from build123d import *

# Parameters (mm, degrees)
F1_DEPTH = 40.386
F2_R     = 15.605309
F3_DEPTH = 61.976


with BuildPart() as f1:
    # F0 (on Top) → F1 (new body)
    with BuildSketch(Plane.XY):
        Polygon((78.89688, 0), (-75.812049, 0), (-75.812049, -32.37997), (78.89688, -38.405467), align=None)
    extrude(amount=F1_DEPTH)

    # F2 (on face) → F3 (join)
    with BuildSketch(Plane.YZ.offset(78.89688)):
        with Locations((-21.061413, 22.759276)):
            Circle(F2_R)
    extrude(amount=F3_DEPTH)


solid = f1.part
Verification items for the finished model (mm, model axes). A direction names the side the tool comes from. Round coordinates to 2 decimals unless told otherwise and drop trailing zeros. Loops run counter-clockwise (first coordinate to the right, second up) from the corner with the lowest first, then second, coordinate; pieces in that order, holes last. Notation, with made-up numbers: (56, -18.75) - (105, -18.75) arc R14 cw to (105, -5.75) - close; hole circle Ø6 at (25, 40). An arc over 180 degrees is marked (long way). Use a Markdown table: item, result. Add a question column.
1. Thickness scan on probe 1 along X at (y, z) = (-21, 2.5); probe 2 along Y at (x, z) = (-33, 33.5); probe 3 along Y at (x, z) = (-43, 18.5). Record the ranges inside material, lowest first. Write a range as [from, to].
2. Section check B-B, the plane z = 26. Record the boundary of the cut face in (x, y).
3. Gauge pin test, flat ends, axial feed: pin 1 (5 mm diameter, centred on x = 104, z = 23.5, fed in from -Y); pin 2 (10 mm diameter, centred on x = -1.5, z = 17.5, fed in from -Y). Record the tip position at first contact, or that the pin passes through.
4. Section check D-D, the plane x = 38.5. Record the boundary of the cut face in (y, z).
5. Section check A-A, the plane y = -18. Record the boundary of the cut face in (x, z), plus the area to 3 significant figures.
6. Section check C-C, the plane x = -37. Record the boundary of the cut face in (y, z).
7. Access from +Z, -Z, +X, -X, +Y, -Y to the whole of each face (thin tool, end or side, straight path). Record for faces 1 (the face through (0.46, -35.35, 19.91)), 2 (the face through (78.897, -19, 6)).
Checks:
| question | item | result |
|---|---|---|
| 1 | probe 1 | x = [-75.81, 78.9] |
| 1 | probe 2 | y = [-34.05, 0] |
| 1 | probe 3 | y = [-33.66, 0] |
| 2 | outline | (-75.81, -32.38) - (78.9, -38.41) - (78.9, -36.33) - (140.87, -36.33) - (140.87, -5.8) - (78.9, -5.8) - (78.9, 0) - (-75.81, 0) - close |
| 3 | pin 1 | stops at y = -36.67 |
| 3 | pin 2 | stops at y = -35.47 |
| 4 | outline | (-36.83, 0) - (0, 0) - (0, 40.39) - (-36.83, 40.39) - close |
| 5 | outline | (-75.81, 0) - (78.9, 0) - (78.9, 7.46) - (140.87, 7.46) - (140.87, 38.06) - (78.9, 38.06) - (78.9, 40.39) - (-75.81, 40.39) - close |
| 5 | area | 8,140 mm^2 |
| 6 | outline | (-33.89, 0) - (0, 0) - (0, 40.39) - (-33.89, 40.39) - close |
| 7 | face 1 | +Z, -Z, -X, -Y |
| 7 | face 2 | +X |
